Can you work these out from the drawing? Everything is in mm from the part's minimum corner. Give positions to 0.01 mm unless a question says otherwise; leave off trailing zeros. Write each loop counter-clockwise with the first axis right and the second up, starting at its lowest first coordinate (ties: lowest second). Pieces come first, ordered by that corner, then holes. Notation, with made-up numbers: (59, 73) - (63, 73) arc R29 ccw to (63, 102) - close; hole circle Ø6 at (50, 3.5). An arc over 180 degrees is marked (long way). Answer in a Markdown table with one row per item.
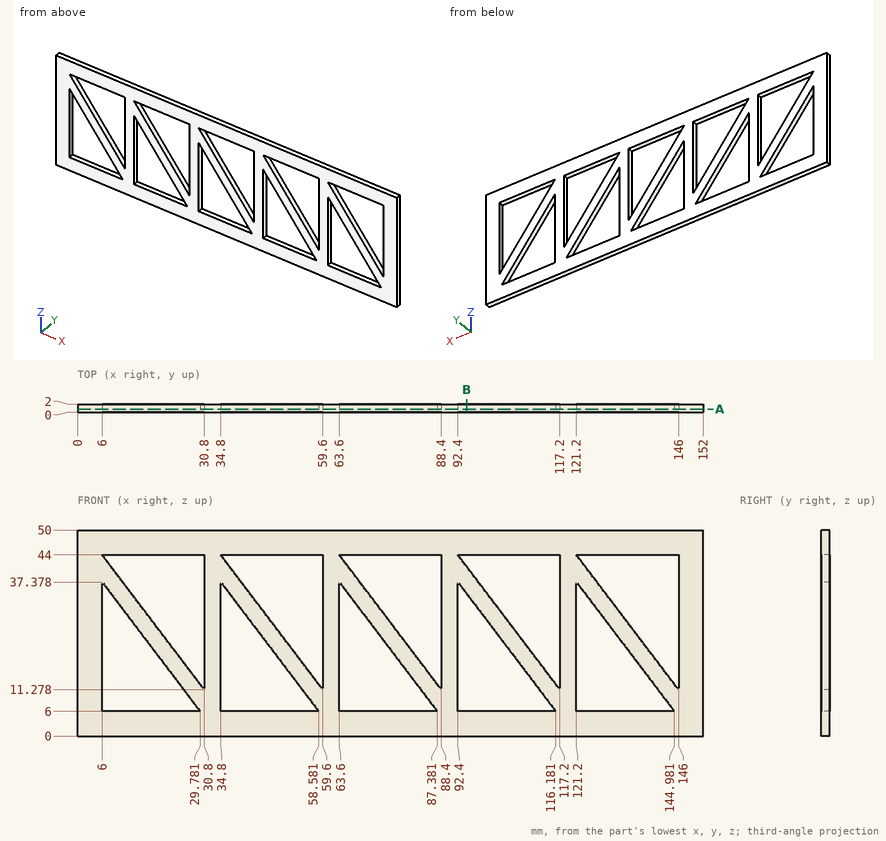
1) Imagine slicing it at A-A (y = 0.75). State how many separate pieces and enclosed holes the cut face has.
Check values:
| item | result |
|---|---|
| separate pieces | 1 |
| enclosed holes | 10 |
2) If I drill on line 1 (Z direction, x = 39, y = 0.65) (1 decimal); line 2 (X direction, y = 0.65, z = 7.5) (1 decimal); line 3 (Z direction, x = 9, y = 1.5), over which ranges is the centre line in solid material (lowest first)?
Check values:
| item | result |
|---|---|
| line 1 | z = 0 to 6, 31.8 to 38.5, 44 to 50 |
| line 2 | x = 0 to 6, 28.6 to 34.8, 57.4 to 63.6, 86.2 to 92.4, 115 to 121.2, 143.8 to 152 |
| line 3 | z = 0 to 6, 33.42 to 40.04, 44 to 50 |
3) Will this pin go through, and if not, where does the flat tip stop? P1, Ø1, axis at y = 0.5, z = 25.5, coming from the -X side.
Check values:
| item | result |
|---|---|
| P1 | stops at x = 0 |
4) Imagine slicing it at B-B (x = 94.5). List the corners of the cut face in (y, z) for me.
Check values:
| item | result |
|---|---|
| outline | (0, 0) - (2, 0) - (2, 6) - (0, 6) - close; (0, 34.61) - (2, 34.61) - (2, 41.23) - (0, 41.23) - close; (0, 44) - (2, 44) - (2, 50) - (0, 50) - close |
